Input: part model. Units: mm. Frame: model coordinates. Give positions to 0.01 mm unless a question says otherwise; leave off trailing zeros. Loops run counter-clockwise (first coordinate to the right, second up) from the corner with the lowest first, then second, coordinate; pieces in that order, holes last. Notation, with made-up numbers: (61.5, 77.5) - (103.5, 77.5) arc R28 cw to (103.5, 96.5) - close; hole circle Ø4 at (52.5, 45.25). An arc over 180 degrees is marked (long way). One line per question, with ' | ' between items. Start each with the question number.
Autodesk Inventor part; units mm, degrees
ref_plane "YZ Plane" through (0, 0, 0) normal (1, 0, 0) x (0, 1, 0)
ref_plane "XZ Plane" through (0, 0, 0) normal (0, 1, 0) x (-1, 0, 0)
ref_plane "XY Plane" through (0, 0, 0) normal (0, 0, 1) x (1, 0, 0)
sketch "Sketch1" plane through (0, 0, 0) normal (0, 1, 0) x (-1, 0, 0)
  line L0 (90, -50) -> (-90, -50)
  line L1 (-90, -50) -> (-90, 50)
  line L2 (-90, 50) -> (90, 50)
  line L3 (90, 50) -> (90, -50)
  line L4 (0, 0) -> (0, -16.1308) construction
  line L5 (0, 0) -> (18.4922, 0) construction
  dimension "d1" = 100
  dimension "d2" = 180
extrude "Extrusion1" add sketch "Sketch1" along normal blind 2.2
sketch "Sketch2" plane through (0, 2.2, 0) normal (0, 1, 0) x (1, 0, 0)
  line L0 (-90, -50) -> (90, -50)
  line L1 (90, -50) -> (90, 50)
  line L2 (90, -50) -> (90, -30)
  line L3 (90, -30) -> (55.6, -30)
  line L4 (55.6, -30) -> (55.6, -50)
  line L5 (55.6, -50) -> (90, -50)
  line L6 (90, -40) -> (55.6, -40) construction
  circle A0 centre (78.8, -40) radius 2.15
  circle A1 centre (72.8, -40) radius 2.15
  circle A2 centre (66.8, -40) radius 2.15
  line L7 (72.8, -40) -> (72.8, -30) construction
  circle A3 centre (72.8, -34) radius 2.15
  circle A4 centre (72.8, -46) radius 2.15
  circle A5 centre (72.8, -40) radius 2.15
  line L8 (0, 0) -> (96.2626, 0) construction
  line L9 (90, 50) -> (90, 30)
  line L10 (90, 30) -> (55.6, 30)
  line L11 (55.6, 30) -> (55.6, 50)
  line L12 (55.6, 50) -> (90, 50)
  line L13 (90, 40) -> (55.6, 40) construction
  circle A6 centre (78.8, 40) radius 2.15
  circle A7 centre (72.8, 40) radius 2.15
  circle A8 centre (66.8, 40) radius 2.15
  line L14 (72.8, 40) -> (72.8, 30) construction
  circle A9 centre (72.8, 34) radius 2.15
  circle A10 centre (72.8, 46) radius 2.15
  circle A11 centre (72.8, 40) radius 2.15
  line L15 (90, 50) -> (-90, 50)
  line L16 (-90, 50) -> (-90, -50)
  line L17 (-48, 40) -> (-72, 40)
  line L18 (-72, 40) -> (-72, 50)
  line L19 (-72, 50) -> (-48, 50)
  line L20 (-48, 50) -> (-48, 40)
  line L21 (-74.3246, 46.5) -> (-4.1674, 46.5) construction
  line L22 (-60, 53.3324) -> (-60, 32.9187) construction
  circle A12 centre (-60, 37.5) radius 2.15
  line L23 (-68.3246, 46.5) -> (1.8326, 46.5) construction
  circle A13 centre (-54, 37.5) radius 2.15
  circle A14 centre (-66, 37.5) radius 2.15
  line L24 (-8.0003, 43.25) -> (-83.9137, 43.25) construction
  circle A15 centre (-78, 43.25) radius 2.15
  circle A16 centre (-84, 43.25) radius 2.15
  circle A17 centre (-42, 43.25) radius 2.15
  circle A18 centre (-36, 43.25) radius 2.15
  line L25 (-48, -40) -> (-72, -40)
  line L26 (-72, -40) -> (-72, -50)
  line L27 (-72, -50) -> (-48, -50)
  line L28 (-48, -50) -> (-48, -40)
  line L29 (-74.3246, -46.5) -> (-4.1674, -46.5) construction
  line L30 (-60, -53.3324) -> (-60, -32.9187) construction
  circle A19 centre (-60, -37.5) radius 2.15
  circle A20 centre (-54, -37.5) radius 2.15
  circle A21 centre (-66, -37.5) radius 2.15
  line L31 (-8.0003, -43.25) -> (-83.9137, -43.25) construction
  circle A22 centre (-78, -43.25) radius 2.15
  circle A23 centre (-84, -43.25) radius 2.15
  circle A24 centre (-36, -43.25) radius 2.15
  circle A25 centre (-42, -43.25) radius 2.15
  circle A26 centre (-60, 37.5) radius 2.5 construction
  dimension "d13" = 20
  dimension "d14" = 34.4
  dimension "d15" = 4.3
  dimension "d16" = 6
  dimension "d17" = 6
  dimension "d18" = 6
  dimension "d27" = 24
  dimension "d28" = 10
  dimension "d29" = 18
  dimension "d31" = 4.3
  dimension "d34" = 6
  dimension "d41" = 6
  dimension "d46" = 6.5
  dimension "d48" = 4.3
  dimension "d49" = 6
  dimension "d52" = 6
  dimension "d60" = 5
extrude "Holes" cut sketch "Sketch2" against normal through all contours A0 | A1 | A2 | A3 | A4 | A6 | A7 | A8 | A9 | A10 | A12 | A13 | A14 | A15 | A16 | A17 | A18 | A19 | A20 | A21 | A22 | A23 | A24 | A25
sketch "Sketch3" plane through (0, 2.2, 0) normal (0, 1, 0) x (1, 0, 0)
  line L0 (33.5, 13.5) -> (-33.5, 13.5) construction
  line L1 (-33.5, 13.5) -> (-33.5, -13.5) construction
  line L2 (-33.5, -13.5) -> (33.5, -13.5) construction
  line L3 (33.5, -13.5) -> (33.5, 13.5) construction
  line L4 (0, 0) -> (39.98, 0) construction
  line L5 (0, 0) -> (0, 21.0122) construction
  circle A0 centre (30, 9) radius 2.15
  circle A1 centre (30, -9) radius 2.15
  circle A2 centre (-30, 9) radius 2.15
  circle A3 centre (-30, -9) radius 2.15
  line L6 (33.5, 7.5) -> (43.5, 7.5)
  line L7 (43.5, 7.5) -> (43.5, -7.5)
  line L8 (43.5, -7.5) -> (33.5, -7.5)
  line L9 (33.5, -7.5) -> (33.5, 7.5)
  dimension "d61" = 67
  dimension "d62" = 27
  dimension "d63" = 4.3
  dimension "d64" = 3.5
  dimension "d65" = 4.5
  dimension "d68" = 10
  dimension "d69" = 15
extrude "Extrusion4" cut sketch "Sketch3" against normal through all
fillet "Fillet1" radius 2 4 edges at (33.5, 1.1, -7.5) (43.5, 1.1, -7.5) (43.5, 1.1, 7.5) (33.5, 1.1, 7.5)
equation "\"d1\" = BodyWidth"
equation "\"d2\" = BodyLength"
equation "\"d3\" = Depth"
equation "\"d15\" = Holes"
equation "\"d27\" = MotorWidth"
equation "\"d31\" = Holes"
equation "\"d57\" = Depth"
equation "\"BodyWidth\" = 100"
equation "\"BodyLength\" = 180"
equation "\"Holes\" = 4.3"
equation "\"Depth\" = 2.2"
equation "\"d20\" = 4.3"
equation "\"MotorWidth\" = 24"
Q1. Section C-C, the plane y = 0.7. Count the separate pieces of the cut face and the enclosed holes in it, plus the area to 3 significant figures.
Q2. Section A-A, the plane x = -42. Output: boundary loops of the cut face in (y, z).
Q3. Line query: L1, parallel to X at y = 2.05, z = -40; L2, parallel to X at y = 1.35, z = -37.5; L3, parallel to Z at x = -36, y = 0.65. Output: solid intervals per line, ascending. Write a range as from..to.
Q4. Section B-B, the plane x = 72.8. Output: boundary loops of the cut face in (y, z), plus the area to 3 significant figures.
Solved:
1) separate pieces: 1 | enclosed holes: 29 | area: 17,400 mm²
2) outline: (0, -50) - (2.2, -50) - (2.2, -45.4) - (0, -45.4) - close; (0, -41.1) - (2.2, -41.1) - (2.2, 41.1) - (0, 41.1) - close; (0, 45.4) - (2.2, 45.4) - (2.2, 50) - (0, 50) - close
3) L1: x = -90..64.65, 68.95..70.65, 74.95..76.65, 80.95..90 | L2: x = -90..-68.15, -63.85..-62.15, -57.85..-56.15, -51.85..90 | L3: z = -50..-45.4, -41.1..41.1, 45.4..50
4) outline: (0, -50) - (2.2, -50) - (2.2, -48.15) - (0, -48.15) - close; (0, -43.85) - (2.2, -43.85) - (2.2, -42.15) - (0, -42.15) - close; (0, -37.85) - (2.2, -37.85) - (2.2, -36.15) - (0, -36.15) - close; (0, -31.85) - (2.2, -31.85) - (2.2, 31.85) - (0, 31.85) - close; (0, 36.15) - (2.2, 36.15) - (2.2, 37.85) - (0, 37.85) - close; (0, 42.15) - (2.2, 42.15) - (2.2, 43.85) - (0, 43.85) - close; (0, 48.15) - (2.2, 48.15) - (2.2, 50) - (0, 50) - close | area: 163 mm²
